For this review, use the dimensioned drawing (mm, ordinates from the lowest corner) and the shaded views. A direction names the side the tool comes from. Coordinates: 2 decimals unless noted, no trailing zeros. Write each loop counter-clockwise with the first axis right and the second up, starting at its lowest first coordinate (ties: lowest second). Pieces come first, ordered by that corner, then holes. Notation, with made-up numbers: M 7,6.25 L 42,6.25 A30 ccw 42,45.25 Z; hole C 15,30.25 d6. An arc over 180 degrees is marked long. Return JSON: item names as keys, results as strings.
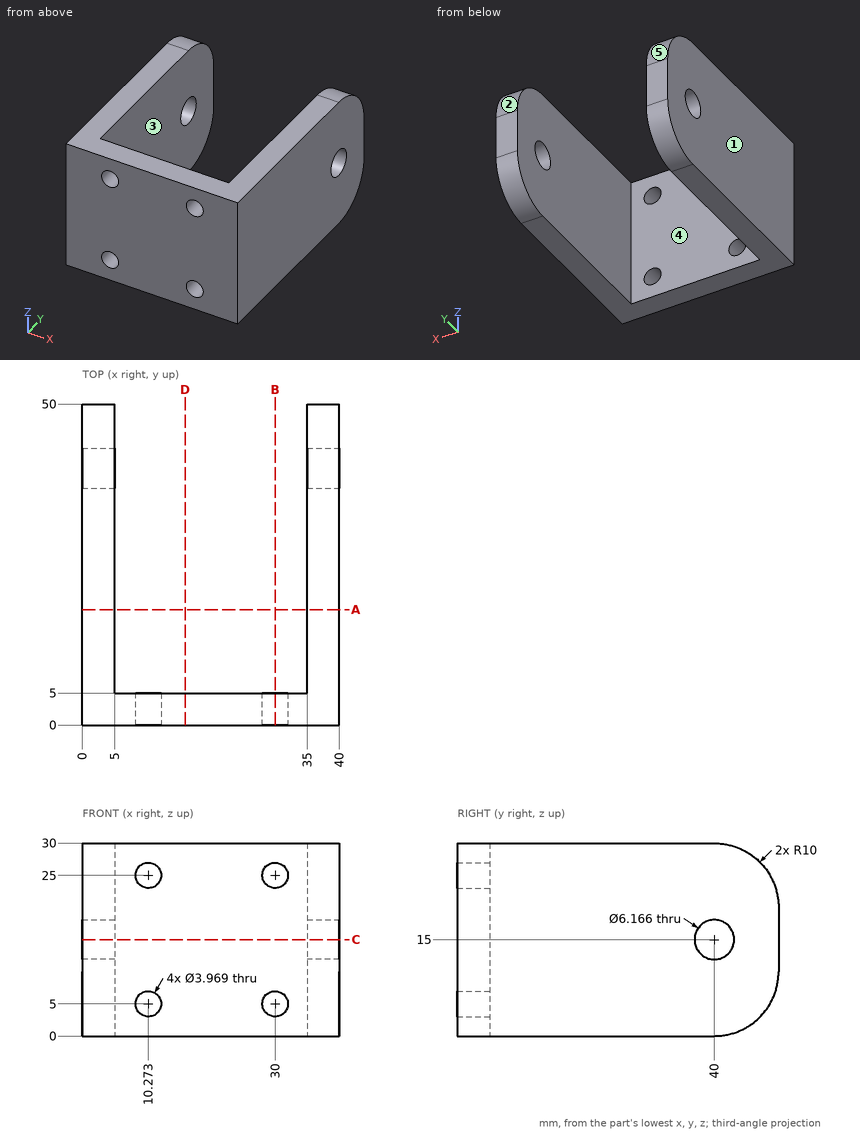
1. We need section D-D (x = 16). State the section outline as (y, z) points.
Checks:
{"outline": "M 0,0 L 5,0 L 5,30 L 0,30 Z"}
2. Clearance check with flat-ended pins moving along their axes: pin 1 Ø3.5 at (x, z) = (10.27, 5) entering from +Y; pin 2 Ø2 at (x, z) = (6.5, 21) entering from +Y. State where each tip first meets the part, or that it passes through.
Checks:
{"pin 1": "through", "pin 2": "y = 5"}
3. We need section B-B (x = 30). State the section outline as (y, z) points.
Checks:
{"outline": "M 0,0 L 5,0 L 5,3.02 L 0,3.02 Z; M 0,6.98 L 5,6.98 L 5,23.02 L 0,23.02 Z; M 0,26.98 L 5,26.98 L 5,30 L 0,30 Z"}
4. We need section A-A (y = 18). State the section outline as (x, z) points.
Checks:
{"outline": "M 0,0 L 5,0 L 5,30 L 0,30 Z; M 35,0 L 40,0 L 40,30 L 35,30 Z"}
5. Draft analysis for pull direction X (two halves, no side actions). For the marked faces 1, 2 and 3, state which applies: +X half, -X half, draft (parallel to the pull), parting line (faces both ways), or undercut.
Checks:
{"face 1": "-X half", "face 2": "draft", "face 3": "undercut"}
6. We need section C-C (z = 15). State the section outline as (x, y) points.
Checks:
{"outline": "M 0,0 L 40,0 L 40,36.92 L 35,36.92 L 35,5 L 5,5 L 5,36.92 L 0,36.92 Z; M 0,43.08 L 5,43.08 L 5,50 L 0,50 Z; M 35,43.08 L 40,43.08 L 40,50 L 35,50 Z"}
7. Wall thickness on L1, parallel to X at y = 2.5, z = 25; L2, parallel to X at y = 44, z = 10.25; L3, parallel to Z at x = 30, y = 2: over which ranges is each line inside the solid? List them lowest first. Write a range as from..to.
Checks:
{"L1": "0..8.29, 12.26..28.02, 31.98..40", "L2": "0..5, 35..40", "L3": "0..3.02, 6.98..23.02, 26.98..30"}
8. For the marked faces 4 and 5, list the 3-axis set-ups (+Z, -Z, +X, -X, +Y, -Y) from which the entire face can be reached by the end or side of a thin tool; tool diameter is ignored.
Checks:
{"face 4": "+Z, -Z, +Y", "face 5": "+Z, +X, -X, +Y"}
